```python
from build123d import *

# Parameters (mm, degrees)
SKETCH1_W               = 190
SKETCH1_H               = 190
BOSS_EXTRUDE1_DEPTH     = 40
SHELL1_T                = 3
FILLET1_R               = 5
SKETCH5_W               = 10
SKETCH5_H               = 10
SKETCH5_R               = 1.6
BOSS_EXTRUDE3_DEPTH     = 37
MIRROR2_COPY_1_SKETCH_W = 10
MIRROR2_COPY_1_SKETCH_H = 10
MIRROR2_COPY_1_SKETCH_R = 1.6
MIRROR2_COPY_1_DEPTH    = 37
FILLET3_R               = 3
SKETCH6_R               = 3.75
SKETCH6_R_2             = 1.6
BOSS_EXTRUDE4_DEPTH     = 7
LPATTERN1_COUNT         = 5
LPATTERN1_PITCH         = 37
SKETCH7_R               = 4
SKETCH7_R_2             = 1.6
BOSS_EXTRUDE5_DEPTH     = 5
SKETCH8_R               = 4
SKETCH8_R_2             = 1.6
BOSS_EXTRUDE6_DEPTH     = 10
LPATTERN2_COUNT         = 2
LPATTERN2_PITCH         = 60


with BuildPart() as part:
    # Sketch1 → Boss-Extrude1 (new body)
    with BuildSketch(Plane(origin=(0, 0, 0), x_dir=(1, 0, 0), z_dir=(0, 1, 0))):
        Rectangle(SKETCH1_W, SKETCH1_H)
    extrude(amount=BOSS_EXTRUDE1_DEPTH)

    # Shell1
    shell1_openings = [part.faces().sort_by_distance(p)[0] for p in [
        (0, 40, 0),
    ]]
    offset(amount=SHELL1_T, openings=shell1_openings, kind=Kind.INTERSECTION)

    # Fillet1
    # the kernel refuses this fillet: 5 mm, written as the material it takes off along each edge
    with BuildSketch(Plane(origin=(-98, 52.5, 98), x_dir=(1, 0, 0), z_dir=(0, -1, 0)), Plane(origin=(98, -15.5, 98), x_dir=(-1, 0, 0), z_dir=(0, 1, 0)), Plane(origin=(98, -15.5, -98), x_dir=(0, 0, 1), z_dir=(0, 1, 0)), Plane(origin=(-98, -15.5, -98), x_dir=(1, 0, 0), z_dir=(0, 1, 0))) as fillet1_piece_1:
        with BuildLine():
            CenterArc((FILLET1_R, -FILLET1_R), FILLET1_R, 90, 90)
            Line((0, -FILLET1_R), (0, 0))
            Line((0, 0), (FILLET1_R, 0))
        make_face()
    extrude(amount=68, mode=Mode.SUBTRACT)

    # Sketch5 → Boss-Extrude3 (add)
    with BuildSketch(Plane(origin=(0, 0, 0), x_dir=(1, 0, 0), z_dir=(0, 1, 0))):
        with Locations((-90, 90)):
            Rectangle(SKETCH5_W, SKETCH5_H)
        with Locations(Location((-90, 90, 0), (0, 0, 270))):
            Circle(SKETCH5_R, mode=Mode.SUBTRACT)
    boss_extrude3 = extrude(amount=BOSS_EXTRUDE3_DEPTH)

    # Mirror1: Boss-Extrude3 across plane
    add(boss_extrude3.mirror(Plane(origin=(0, 0, 0), x_dir=(0, 0, 1), z_dir=(1, 0, 0))))

    # Mirror2: Boss-Extrude3 across plane
    add(boss_extrude3.mirror(Plane.XY))

    # Mirror2 copy 1 sketch → Mirror2 copy 1 (add)
    with BuildSketch(Plane(origin=(0, 0, 0), x_dir=(-1, 0, 0), z_dir=(0, 1, 0))):
        with Locations((-90, 90)):
            Rectangle(MIRROR2_COPY_1_SKETCH_W, MIRROR2_COPY_1_SKETCH_H)
        with Locations(Location((-90, 90, 0), (0, 0, 270))):
            Circle(MIRROR2_COPY_1_SKETCH_R, mode=Mode.SUBTRACT)
    extrude(amount=MIRROR2_COPY_1_DEPTH)

    # Fillet3
    fillet3_edges = [part.edges().sort_by_distance(p)[0] for p in [
        (-95, 18.5, 85),
        (-85, 18.5, 95),
        (-85, 18.5, 85),
        (-95, 18.5, -85),
        (-85, 18.5, -85),
        (-85, 18.5, -95),
        (95, 18.5, -85),
        (85, 18.5, -95),
        (85, 18.5, -85),
        (95, 18.5, 85),
        (85, 18.5, 85),
        (85, 18.5, 95),
    ]]
    fillet(fillet3_edges, radius=FILLET3_R)

    # Sketch6 → Boss-Extrude4 (add)
    # profile 1 of 4: a face of its own
    with BuildSketch(Plane(origin=(0, -3, 0), x_dir=(1, 0, 0), z_dir=(0, 1, 0))):
        with Locations(Location((-65, 15.4, 0), (0, 0, 90))):
            Circle(SKETCH6_R)
        with Locations(Location((-65, 15.4, 0), (0, 0, 90))):
            Circle(SKETCH6_R_2, mode=Mode.SUBTRACT)
    # profile 2 of 4: a face of its own
    with BuildSketch(Plane(origin=(0, -3, 0), x_dir=(1, 0, 0), z_dir=(0, 1, 0))):
        with Locations(Location((-65, -10, 0), (0, 0, 90))):
            Circle(SKETCH6_R)
        with Locations(Location((-65, -10, 0), (0, 0, 90))):
            Circle(SKETCH6_R_2, mode=Mode.SUBTRACT)
    # profile 3 of 4: a face of its own
    with BuildSketch(Plane(origin=(0, -3, 0), x_dir=(1, 0, 0), z_dir=(0, 1, 0))):
        with Locations(Location((-82.8, 15.4, 0), (0, 0, 90))):
            Circle(SKETCH6_R)
        with Locations(Location((-82.8, 15.4, 0), (0, 0, 90))):
            Circle(SKETCH6_R_2, mode=Mode.SUBTRACT)
    # profile 4 of 4: a face of its own
    with BuildSketch(Plane(origin=(0, -3, 0), x_dir=(1, 0, 0), z_dir=(0, 1, 0))):
        with Locations(Location((-82.8, -10, 0), (0, 0, 90))):
            Circle(SKETCH6_R)
        with Locations(Location((-82.8, -10, 0), (0, 0, 90))):
            Circle(SKETCH6_R_2, mode=Mode.SUBTRACT)
    boss_extrude4 = extrude(amount=BOSS_EXTRUDE4_DEPTH)

    # LPattern1: Boss-Extrude4 ×5
    with Locations(*[(i * LPATTERN1_PITCH, 0, 0) for i in range(1, LPATTERN1_COUNT)]):
        add(boss_extrude4)

    # Sketch7 → Boss-Extrude5 (add)
    # profile 1 of 4: a face of its own
    with BuildSketch(Plane(origin=(0, 0, 0), x_dir=(1, 0, 0), z_dir=(0, 1, 0))):
        with Locations(Location((-90, -29.2, 0), (0, 0, 90))):
            Circle(SKETCH7_R)
        with Locations(Location((-90, -29.2, 0), (0, 0, 270))):
            Circle(SKETCH7_R_2, mode=Mode.SUBTRACT)
    # profile 2 of 4: a face of its own
    with BuildSketch(Plane(origin=(0, 0, 0), x_dir=(1, 0, 0), z_dir=(0, 1, 0))):
        with Locations(Location((-90, -80, 0), (0, 0, 90))):
            Circle(SKETCH7_R)
        with Locations(Location((-90, -80, 0), (0, 0, 270))):
            Circle(SKETCH7_R_2, mode=Mode.SUBTRACT)
    # profile 3 of 4: a face of its own
    with BuildSketch(Plane(origin=(0, 0, 0), x_dir=(1, 0, 0), z_dir=(0, 1, 0))):
        with Locations(Location((70, -80, 0), (0, 0, 90))):
            Circle(SKETCH7_R)
        with Locations(Location((70, -80, 0), (0, 0, 270))):
            Circle(SKETCH7_R_2, mode=Mode.SUBTRACT)
    # profile 4 of 4: a face of its own
    with BuildSketch(Plane(origin=(0, 0, 0), x_dir=(1, 0, 0), z_dir=(0, 1, 0))):
        with Locations(Location((70, -29.2, 0), (0, 0, 90))):
            Circle(SKETCH7_R)
        with Locations(Location((70, -29.2, 0), (0, 0, 270))):
            Circle(SKETCH7_R_2, mode=Mode.SUBTRACT)
    extrude(amount=BOSS_EXTRUDE5_DEPTH)

    # Sketch8 → Boss-Extrude6 (add)
    # profile 1 of 4: a face of its own
    with BuildSketch(Plane(origin=(0, 0, 0), x_dir=(1, 0, 0), z_dir=(0, 1, 0))):
        with Locations(Location((-31.74, 37.93, 0), (0, 0, 90))):
            Circle(SKETCH8_R)
        with Locations(Location((-31.74, 37.93, 0), (0, 0, 270))):
            Circle(SKETCH8_R_2, mode=Mode.SUBTRACT)
    # profile 2 of 4: a face of its own
    with BuildSketch(Plane(origin=(0, 0, 0), x_dir=(1, 0, 0), z_dir=(0, 1, 0))):
        with Locations(Location((-36.82, 90, 0), (0, 0, 90))):
            Circle(SKETCH8_R)
        with Locations(Location((-36.82, 90, 0), (0, 0, 270))):
            Circle(SKETCH8_R_2, mode=Mode.SUBTRACT)
    # profile 3 of 4: a face of its own
    with BuildSketch(Plane(origin=(0, 0, 0), x_dir=(1, 0, 0), z_dir=(0, 1, 0))):
        with Locations(Location((-80, 39.2, 0), (0, 0, 90))):
            Circle(SKETCH8_R)
        with Locations(Location((-80, 39.2, 0), (0, 0, 270))):
            Circle(SKETCH8_R_2, mode=Mode.SUBTRACT)
    # profile 4 of 4: a face of its own
    with BuildSketch(Plane(origin=(0, 0, 0), x_dir=(1, 0, 0), z_dir=(0, 1, 0))):
        with Locations(Location((-64.76, 90, 0), (0, 0, 90))):
            Circle(SKETCH8_R)
        with Locations(Location((-64.76, 90, 0), (0, 0, 270))):
            Circle(SKETCH8_R_2, mode=Mode.SUBTRACT)
    boss_extrude6 = extrude(amount=BOSS_EXTRUDE6_DEPTH)

    # LPattern2: Boss-Extrude6 ×2
    with Locations(*[(i * LPATTERN2_PITCH, 0, 0) for i in range(1, LPATTERN2_COUNT)]):
        add(boss_extrude6)


solid = part.part
```
The listing builds one solid part. Answer for the finished solid, in the listing's coordinates (mm). A direction names the side the tool comes from. Give positions to 0.01 mm unless a question says otherwise; leave off trailing zeros. Order: outer loops, then holes, each group sorted by start corner. A loop starts at its lowest first (then second) coordinate and runs counter-clockwise, first axis right, second up.
1) Given P1, Ø2.5, axis at x = 65.2, z = -15.4, coming from the +Y side; P2, Ø4, axis at x = -38, z = -92, coming from the +Y side; P3, Ø8, axis at x = -28, z = 11.5, coming from the +Y side, each flat-ended and moving along its own axis, determine where each tip first touches the part or whether it passes through.
Reported:
P1: stops at y = 0
P2: stops at y = 10
P3: stops at y = 4
2) Find section A-A on x = 52. Write down the section's boundary in (y, z), then the cut area to 3 significant figures.
Reported:
outline: (-3, -98) - (40, -98) - (40, -95) - (0, -95) - (0, 95) - (40, 95) - (40, 98) - (-3, 98) - close
area: 828 mm2
3) For faces 4 (the face through (-40.786, 4.93, -89.479)), 5 (the face through (96, 18, 97)), determine the directions among +Z, -Z, +X, -X, +Y, -Y from which every point of the face is accessible in a straight line to the end or side of a thin tool.
Reported:
face 4: +Y
face 5: +Z, +X, +Y, -Y
4) Determine the mould class of faces 1 (the face through (-27.835, 4.93, -37.063)), 2 (the face through (98, 18, 1)), 3 (the face through (97, 18, -96)) for opening direction Z: pulls with the +Z half, pulls with the -Z half, needs draft (parallel to the pull), parting line crosses it, or undercut.
Reported:
face 1: undercut
face 2: needs draft
face 3: pulls with the -Z half
5) Consider line 1 along Z through (x, y) = (-4.76, 8); line 2 along X through (y, z) = (27, -90); line 3 along Z through (x, y) = (70, 3.7). Determine where each line is inside the solid, lowest interval first.
Reported:
line 1: z = -98 to -95, -94 to -91.6, -88.4 to -86, 95 to 98
line 2: x = -98 to -91.6, -88.4 to -85, 85 to 88.4, 91.6 to 98
line 3: z = -98 to -95, 25.2 to 27.6, 30.8 to 33.2, 76 to 78.4, 81.6 to 84, 95 to 98
6) Find section B-B on y = 30. Give the number of separate pieces and of enclosed holes in the cut face, then the cut area to 3 significant figures.
Reported:
separate pieces: 1
enclosed holes: 5
area: 2,670 mm2
